Verification items for the finished model (mm, model axes). A direction names the side the tool comes from. Coordinates: 2 decimals unless noted, no trailing zeros. Loops run counter-clockwise (first coordinate to the right, second up) from the corner with the lowest first, then second, coordinate; pieces in that order, holes last. Notation, with made-up numbers: (-27, 70) -> (-2, 70) arc R5 cw to (-2, 78) -> close; hole circle Ø3 at (-36, 20.5). An arc over 180 degrees is marked (long way). Write item = value, one per line.
Autodesk Inventor part; units mm, degrees
ref_plane "YZ Plane" through (0, 0, 0) normal (1, 0, 0) x (0, 1, 0)
ref_plane "XZ Plane" through (0, 0, 0) normal (0, 1, 0) x (-1, 0, 0)
ref_plane "XY Plane" through (0, 0, 0) normal (0, 0, 1) x (1, 0, 0)
sketch "スケッチ1" plane through (0, 0, 0) normal (0, 0, 1) x (1, 0, 0)
  line L0 (4.5, -4.5) -> (-4.5, -4.5)
  line L1 (-4.5, -4.5) -> (-4.5, 4.5)
  line L2 (-4.5, 4.5) -> (4.5, 4.5)
  line L3 (4.5, 4.5) -> (4.5, -4.5)
  line L4 (4.5, -4.5) -> (-4.5, 4.5) construction
  line L5 (-4.5, -4.5) -> (4.5, 4.5) construction
  line L6 (3.5, 3.5) -> (-3.5, 3.5)
  line L7 (-3.5, 3.5) -> (-3.5, -3.5)
  line L8 (-3.5, -3.5) -> (3.5, -3.5)
  line L9 (3.5, -3.5) -> (3.5, 3.5)
  point P0 (0, 0)
  dimension "d0" = 9
  dimension "d1" = 9
  dimension "d2" = 1
extrude "押し出し1" add sketch "スケッチ1" along normal blind 52
sketch "スケッチ3" plane through (4.5, -4.5, 0) normal (1, 0, 0) x (0, 0, -1)
  line L0 (0, 9) -> (0, 0)
  line L1 (0, 9) -> (-52, 9)
  line L2 (-52, 0) -> (-52, 9)
  line L3 (0, 0) -> (-52, 0)
  line L4 (-52, 4.5) -> (0, 4.5) construction
  line L5 (-26, 4.5) -> (-26, 9) construction
  circle A0 centre (-47, 4.5) radius 1.6
  circle A1 centre (-5, 4.5) radius 1.6
  dimension "d9" = 3.2
  dimension "d10" = 5
extrude "押し出し3" cut sketch "スケッチ3" against normal through all contours A0 | A1
sketch "スケッチ4" plane through (-4.5, -4.5, 0) normal (0, -1, 0) x (1, 0, 0)
  line L0 (9, 0) -> (0, 0)
  line L1 (9, 0) -> (9, 52)
  line L2 (0, 52) -> (9, 52)
  line L3 (0, 0) -> (0, 52)
  line L4 (9, 48.6) -> (9, 45.4)
  line L5 (8, 45.4) -> (8, 48.6)
  line L6 (0, 48.6) -> (0, 45.4)
  line L7 (1, 48.6) -> (1, 45.4)
  line L8 (9, 6.6) -> (9, 3.4)
  line L9 (8, 3.4) -> (8, 6.6)
  line L10 (1, 6.6) -> (1, 3.4)
  line L11 (4.5, 52) -> (4.5, 0) construction
  line L12 (9, 45.4) -> (0, 45.4)
  circle A0 centre (4.5, 40.4) radius 1.6
  line L13 (9, 26) -> (0, 26) construction
  circle A1 centre (4.5, 11.6) radius 1.6
  dimension "d13" = 3.2
  dimension "d14" = 5
  dimension "d15" = 4.5
extrude "押し出し4" cut sketch "スケッチ4" against normal through all contours A0 | A1
properties part number "型" material "アルミニウム 2014-T6"
1) Sectioned sample at D-D, the plane x = 2.25. Record the cut outline in (y, z), plus the area to 3 significant figures.
Ans:
outline = (-4.5, 0) -> (-3.5, 0) -> (-3.5, 52) -> (-4.5, 52) -> close; (3.5, 0) -> (4.5, 0) -> (4.5, 52) -> (3.5, 52) -> close
area = 104 mm2
2) Sectioned sample at C-C, the plane z = 47. Record the cut outline in (x, y).
Ans:
outline = (-4.5, -4.5) -> (4.5, -4.5) -> (4.5, -1.6) -> (3.5, -1.6) -> (3.5, -3.5) -> (-3.5, -3.5) -> (-3.5, -1.6) -> (-4.5, -1.6) -> close; (-4.5, 1.6) -> (-3.5, 1.6) -> (-3.5, 3.5) -> (3.5, 3.5) -> (3.5, 1.6) -> (4.5, 1.6) -> (4.5, 4.5) -> (-4.5, 4.5) -> close
3) Sectioned sample at B-B, the plane y = 0. Record the cut outline in (x, z), plus the area to 3 significant figures.
Ans:
outline = (-4.5, 0) -> (-3.5, 0) -> (-3.5, 3.4) -> (-4.5, 3.4) -> close; (-4.5, 6.6) -> (-3.5, 6.6) -> (-3.5, 45.4) -> (-4.5, 45.4) -> close; (-4.5, 48.6) -> (-3.5, 48.6) -> (-3.5, 52) -> (-4.5, 52) -> close; (3.5, 0) -> (4.5, 0) -> (4.5, 3.4) -> (3.5, 3.4) -> close; (3.5, 6.6) -> (4.5, 6.6) -> (4.5, 45.4) -> (3.5, 45.4) -> close; (3.5, 48.6) -> (4.5, 48.6) -> (4.5, 52) -> (3.5, 52) -> close
area = 91.2 mm2
4) Sectioned sample at A-A, the plane x = 0. Record the cut outline in (y, z), plus the area to 3 significant figures.
Ans:
outline = (-4.5, 0) -> (-3.5, 0) -> (-3.5, 10) -> (-4.5, 10) -> close; (-4.5, 13.2) -> (-3.5, 13.2) -> (-3.5, 38.8) -> (-4.5, 38.8) -> close; (-4.5, 42) -> (-3.5, 42) -> (-3.5, 52) -> (-4.5, 52) -> close; (3.5, 0) -> (4.5, 0) -> (4.5, 10) -> (3.5, 10) -> close; (3.5, 13.2) -> (4.5, 13.2) -> (4.5, 38.8) -> (3.5, 38.8) -> close; (3.5, 42) -> (4.5, 42) -> (4.5, 52) -> (3.5, 52) -> close
area = 91.2 mm2
5) Material ranges on line 1 (Z direction, x = 0, y = 4.05); line 2 (X direction, y = 1.25, z = 32), recorded low to high.
Ans:
line_1 = 0 to 10, 13.2 to 38.8, 42 to 52
line_2 = -4.5 to -3.5, 3.5 to 4.5
6) Tool access check on faces 1 (the face through (0, 3.5, 26)), 2 (the face through (-4, 0, 52)). Record the directions out of +Z, -Z, +X, -X, +Y, -Y that give a thin tool (end or side, any length) a straight path to the whole face; none if there is none.
Ans:
face_1 = +Z, -Z
face_2 = +Z, +X, -X, +Y, -Y
7) Release check for a two-part mould opening along X. For faces 3 (the face through (-3.993, 0.481, 45.474)), 4 (the face through (0, -4, 10)), 5 (the face through (4.5, 0, 26)), 6 (the face through (0, -3.5, 26)) record: pulls with the +X half, pulls with the -X half, needs draft (parallel to the pull), parting line crosses it, or undercut.
Ans:
face_3 = needs draft
face_4 = undercut
face_5 = pulls with the +X half
face_6 = undercut
